Read the model definition and answer for the solid it produces. Units are mm, in the model's axes. A direction names the side the tool comes from. Coordinates: 2 decimals unless noted, no trailing zeros. Loops run counter-clockwise (first coordinate to the right, second up) from the corner with the lowest first, then second, coordinate; pieces in that order, holes last. Notation, with made-up numbers: M -1,-9.5 L 14,-9.5 A26 ccw 14,22.5 Z; hole C 53.25,47 d1. An arc over 180 degrees is marked long. One line per item, written item: value. Start each with the question number.
1. Determine the mould class of faces 4 (the face through (-19.149, -0.014, -45.115)), 5 (the face through (20.651, -0.014, -45.115)), 6 (the face through (17, 6, 23.5)) for opening direction X: +X half, -X half, draft (parallel to the pull), parting line (faces both ways), or undercut.
2. The part is cut by section B-B (z = -47.5). Write down the section's boundary in (x, y).
3. For faces 1 (the face through (17, 6, 40.5)), 2 (the face through (17, -6, 23.5)), 3 (the face through (-18, 6, 42.5)), determine the directions among +Z, -Z, +X, -X, +Y, -Y from which every point of the face is accessible in a straight line to the end or side of a thin tool.
4. The part is cut by section A-A (y = 3.75). Write down the section's boundary in (x, z).
5. Consider probe 1 along X at (y, z) = (0.25, -47.5); probe 2 along Z at (x, y) = (-18, -7.75); probe 3 along Y at (x, z) = (-2, 46.5). Determine where each line is inside the solid, lowest interval first.
6. Flat-ended cylindrical pins translate along their axes: pin 1 (2 mm diameter, centred on y = -8, z = 24, fed in from +X); pin 2 (1.5 mm diameter, centred on x = -9, z = -32.5, fed in from +Y); pin 3 (7 mm diameter, centred on x = 20, y = -8.5, fed in from -Z); pin 4 (6 mm diameter, centred on x = -16.5, y = -3.5, fed in from +Z). Find the tip coordinate at first contact, or state that the pin passes through.
7. The part is cut by section D-D (x = 3). Write down the section's boundary in (y, z).
```python
from build123d import *

# Parameters (mm, degrees)
SKETCH1_R           = 2.5
BOSS_EXTRUDE1_DEPTH = 1
SKETCH2_W           = 20
SKETCH2_H           = 2
BOSS_EXTRUDE2_DEPTH = 10
FILLET2_R           = 1
FILLET3_R           = 1


with BuildPart() as part:
    # Sketch1 → Boss-Extrude1 (new, symmetric)
    with BuildSketch(Plane(origin=(0, 0, 0), x_dir=(1, 0, 0), z_dir=(0, 1, 0))):
        Polygon((1, 62.5), (34.9, 62.5), (34.9, -62.5), (-34.9, -62.5), (-34.9, 62.5), (-1, 62.5), (-1, 2.5), (1, 2.5), align=None)
        with Locations(Location((-19.9, 47.5, 0), (0, 0, 270))):
            Circle(SKETCH1_R, mode=Mode.SUBTRACT)
        with Locations(Location((19.9, 47.5, 0), (0, 0, 270))):
            Circle(SKETCH1_R, mode=Mode.SUBTRACT)
    extrude(amount=BOSS_EXTRUDE1_DEPTH, both=True)

    # Sketch2 → Boss-Extrude2 (add)
    with BuildSketch(Plane(origin=(0, 1, 0), x_dir=(1, 0, 0), z_dir=(0, 1, 0))):
        with Locations((17.4, -24.5)):
            Rectangle(SKETCH2_W, SKETCH2_H)
        with Locations((17.4, -41.5)):
            Rectangle(SKETCH2_W, SKETCH2_H)
        with Locations((-17.4, -41.5)):
            Rectangle(SKETCH2_W, SKETCH2_H)
        with Locations((-17.4, -24.5)):
            Rectangle(SKETCH2_W, SKETCH2_H)
    boss_extrude2 = extrude(amount=BOSS_EXTRUDE2_DEPTH)

    # Mirror1: Boss-Extrude2 across plane
    add(boss_extrude2.mirror(Plane.ZX))

    # Fillet2
    fillet2_edges = [part.edges().sort_by_distance(p)[0] for p in [
        (7.4, -1, 24.5),
        (17.4, -1, 25.5),
        (27.4, -1, 24.5),
        (17.4, -1, 23.5),
        (7.4, -1, 41.5),
        (17.4, -1, 42.5),
        (27.4, -1, 41.5),
        (17.4, -1, 40.5),
        (-7.4, -1, 41.5),
        (-17.4, -1, 40.5),
        (-27.4, -1, 41.5),
        (-17.4, -1, 42.5),
        (-17.4, -1, 23.5),
        (-27.4, -1, 24.5),
        (-17.4, -1, 25.5),
        (-7.4, -1, 24.5),
    ]]
    fillet(fillet2_edges, radius=FILLET2_R)

    # Fillet3
    fillet3_edges = [part.edges().sort_by_distance(p)[0] for p in [
        (7.4, 1, 24.5),
        (17.4, 1, 25.5),
        (27.4, 1, 24.5),
        (17.4, 1, 23.5),
        (7.4, 1, 41.5),
        (17.4, 1, 42.5),
        (27.4, 1, 41.5),
        (17.4, 1, 40.5),
        (-7.4, 1, 41.5),
        (-17.4, 1, 40.5),
        (-27.4, 1, 41.5),
        (-17.4, 1, 42.5),
        (-17.4, 1, 23.5),
        (-27.4, 1, 24.5),
        (-17.4, 1, 25.5),
        (-7.4, 1, 24.5),
    ]]
    fillet(fillet3_edges, radius=FILLET3_R)


solid = part.part
```
Answer block:
1. face 4: undercut
1. face 5: undercut
1. face 6: draft
2. outline: M -34.9,-1 L -22.4,-1 L -22.4,1 L -34.9,1 Z; M -17.4,-1 L -1,-1 L -1,1 L -17.4,1 Z; M 1,-1 L 17.4,-1 L 17.4,1 L 1,1 Z; M 22.4,-1 L 34.9,-1 L 34.9,1 L 22.4,1 Z
3. face 1: +X, -X, +Y
3. face 2: -Z, +X, -X, -Y
3. face 3: +Z, +X, -X, +Y
4. outline: M -27.4,23.5 L -7.4,23.5 L -7.4,25.5 L -27.4,25.5 Z; M -27.4,40.5 L -7.4,40.5 L -7.4,42.5 L -27.4,42.5 Z; M 7.4,23.5 L 27.4,23.5 L 27.4,25.5 L 7.4,25.5 Z; M 7.4,40.5 L 27.4,40.5 L 27.4,42.5 L 7.4,42.5 Z
5. probe 1: x = -34.9 to -22.4, -17.4 to -1, 1 to 17.4, 22.4 to 34.9
5. probe 2: z = 23.5 to 25.5, 40.5 to 42.5
5. probe 3: y = -1 to 1
6. pin 1: stops at x = 27.4
6. pin 2: stops at y = 1
6. pin 3: stops at z = 23.5
6. pin 4: stops at z = 62.5
7. outline: M -1,-62.5 L 1,-62.5 L 1,62.5 L -1,62.5 Z
